Work out the finished part from the listing and answer in its coordinate system (mm). Face numbers are marked on the shaded views. A direction names the side the tool comes from. Coordinates: 2 decimals unless noted, no trailing zeros. Loops run counter-clockwise (first coordinate to the right, second up) from the corner with the lowest first, then second, coordinate; pieces in that order, holes last. Notation, with made-up numbers: (34, 20.25) - (91, 20.25) arc R26 ccw to (91, 57.25) - close; hole circle Ø11 at (4, 61). An arc over 180 degrees is marked (long way). Write each question's results on one line, items separated by ' | '. Start each with the question number.
Item 1: Consider probe 1 along Z at (x, y) = (11, -5); probe 2 along Z at (x, y) = (50.5, -19); probe 3 along Z at (x, y) = (7.5, -9.5). Determine where each line is inside the solid, lowest interval first. Write a range as [from, to].
Item 2: Each of these flat-tipped pins is pushed along its axis until it touches: pin 1 Ø5.5 at (x, y) = (8, -12) entering from -Z; pin 2 Ø6 at (x, y) = (28.5, 0.5) entering from +Z; pin 3 Ø4 at (y, z) = (-1, 0) entering from +X. Where does it stop, or does it pass through?
Item 3: A tool of negligible diameter and unlimited length cuts with its end or side. For the marked faces 4 and 5, from which of +Z, -Z, +X, -X, +Y, -Y can it reach the whole face along a straight path? Write none if from no direction.
Item 4: For a pull along X with two mould halves and no side action, classify the marked faces 1, 2 and 3 as +X half, -X half, draft (parallel to the pull), parting line (faces both ways), or undercut.
Item 5: Section A-A, the plane x = 18 is taken. Write down the section's boundary in (y, z).
from build123d import *

# Parameters (mm, degrees)
EXTRUDE_THIN1_DEPTH = 100
CUT_EXTRUDE2_DEPTH  = 33.5
FILLET1_R           = 3
SKETCH6_W           = 108.67085681690114
SKETCH6_H           = 17.87977423217149
CUT_EXTRUDE3_DEPTH  = 166
BOSS_EXTRUDE1_DEPTH = 10.5
CUT_EXTRUDE4_DEPTH  = 27.00000000000001
SKETCH11_R          = 1.749999999999997
CUT_EXTRUDE5_DEPTH  = 5
BOSS_EXTRUDE2_DEPTH = 7.500000000000001
CUT_EXTRUDE6_START  = -15.000000000000002
CUT_EXTRUDE6_DEPTH  = 15.000000000000002
FILLET3_R           = 2
CUT_EXTRUDE7_DEPTH  = 5.000000000000001
FILLET5_R           = 12


with BuildPart() as part:
    # Sketch1 → Extrude-Thin1 (new body)
    with BuildSketch(Plane(origin=(0, 0, 0), x_dir=(0, 0, -1), z_dir=(1, 0, 0))):
        with BuildLine():
            Line((44.99999999999999, -32), (45, -18.000000000000004))
            ThreePointArc((45, -18.000000000000004), (32.040658090715816, -6.957616725901104), (16.501342127994352, -3.94e-15))
            ThreePointArc((16.501342127994352, -3.94e-15), (-9.68e-15, 1.9727576042150758), (-16.501342127994352, 2.58e-15))
            ThreePointArc((-16.501342127994352, 2.58e-15), (-32.040658090715816, -6.957616725901083), (-45, -17.99999999999999))
            Line((-45, -17.99999999999999), (-45.00000000000001, -31.999999999999986))
            Line((-45.00000000000001, -31.999999999999986), (-48.00000000000001, -31.999999999999986))
            Line((-48.00000000000001, -31.999999999999986), (-48, -16.881858139762553))
            ThreePointArc((-48, -16.881858139762553), (-34.09998293164343, -4.712774745757805), (-17.2676846598946, 2.901081047578947))
            ThreePointArc((-17.2676846598946, 2.901081047578947), (-9.055e-14, 4.972757604215076), (17.26768465989443, 2.901081047578978))
            ThreePointArc((17.26768465989443, 2.901081047578978), (34.099982931643346, -4.71277474575777), (48, -16.881858139762553))
            Line((48, -16.881858139762553), (47.99999999999999, -32))
            Line((47.99999999999999, -32), (44.99999999999999, -32))
        make_face()
    extrude(amount=EXTRUDE_THIN1_DEPTH)

    # Sketch5 → Cut-Extrude2 (cut, symmetric)
    with BuildSketch(Plane(origin=(0, 0, 0), x_dir=(1, 0, 0), z_dir=(0, 1, 0))):
        with BuildLine():
            Line((74.78082212000585, 2.9999999999999996), (74.78082212000585, -3.0000000000000004))
            add(Edge.make_bspline(
                [(74.78082212000585, -3.0000000000000004), (97.6340902919286, -10.562952056895462), (100, -44)],
                knots=[0, 0, 0, 1, 1, 1], degree=2))
            Line((100, -44), (100, 44))
            add(Edge.make_bspline(
                [(74.78082212000585, 2.9999999999999996), (97.6340902919286, 10.562952056895462), (100, 44)],
                knots=[0, 0, 0, 1, 1, 1], degree=2))
        make_face()
    extrude(amount=CUT_EXTRUDE2_DEPTH, both=True, mode=Mode.SUBTRACT)

    # Fillet1
    fillet1_edges = [part.edges().sort_by_distance(p)[0] for p in [
        (50, -16.881858139762556, -48),
        (50, -16.88185813976255, 48),
        (74.78082212000585, 3.4097650316477264, 3.0000000000000004),
        (74.78082212000585, 3.4097650316477246, -2.9999999999999996),
        (46.32817175668929, 2.9010810475789732, -17.267684659894428),
        (46.328171756689336, 2.9010810475789484, 17.267684659894588),
    ]]
    fillet(fillet1_edges, radius=FILLET1_R)

    # Sketch6 → Cut-Extrude3 (cut)
    with BuildSketch(Plane(origin=(0, -2.379e-14, -48.00000000000001), x_dir=(-1, 0, 0), z_dir=(0, -5e-16, -1))):
        with Locations((-40.66457159154943, -32.93988711608573)):
            Rectangle(SKETCH6_W, SKETCH6_H)
    extrude(amount=-CUT_EXTRUDE3_DEPTH, mode=Mode.SUBTRACT)

    # Sketch8 → Boss-Extrude1 (add, symmetric)
    with BuildSketch(Plane.XY):
        Polygon((0, 1.9727576042150723), (-2.8489105039621805, -17.99999999999999), (7.1510894960378195, -17.99999999999999), (15, 1.972757604215074), align=None)
    extrude(amount=BOSS_EXTRUDE1_DEPTH, both=True)

    # Sketch10 → Cut-Extrude4 (cut)
    with BuildSketch(Plane.XY.offset(10.5)):
        with BuildLine():
            Line((-0.3489105039621806, -17.99999999999999), (3.9871579959635945, -17.99999999999999))
            ThreePointArc((3.9871579959635945, -17.99999999999999), (1.8191237460007066, -14.255159652410038), (-0.3489105039621806, -17.99999999999999))
        make_face()
    extrude(amount=-CUT_EXTRUDE4_DEPTH, mode=Mode.SUBTRACT)

    # Sketch11 → Cut-Extrude5 (cut)
    with BuildSketch(Plane(origin=(0, -2.379e-14, -48.00000000000001), x_dir=(-1, 0, 0), z_dir=(0, -5e-16, -1))):
        with Locations(Location((-95, -18.99999999999998, 0), (0, 0, 34.849904579))):
            Circle(SKETCH11_R)
    cut_extrude5 = extrude(amount=-CUT_EXTRUDE5_DEPTH, mode=Mode.SUBTRACT)

    # Mirror1: Cut-Extrude5 across plane
    add(cut_extrude5.mirror(Plane.XY), mode=Mode.SUBTRACT)

    # Sketch12 → Boss-Extrude2 (add, symmetric)
    with BuildSketch(Plane.XY):
        Polygon((74.78082212000585, 1.9727576042150723), (74.78082212000585, -15.901753636370586), (83.21987044067507, -15.901753636370586), (83.21987044067507, -19.589110757152636), (67.6773818593807, -19.589110757152636), (67.6773818593807, 1.9727576042150723), align=None)
    extrude(amount=BOSS_EXTRUDE2_DEPTH, both=True)

    # Sketch13 → Cut-Extrude6 (cut)
    with BuildSketch(Plane(origin=(74.78082212000585, 0, 0), x_dir=(0, 0, -1), z_dir=(1, 0, 0)).offset(CUT_EXTRUDE6_START)):
        with BuildLine():
            Line((-7.500000000000001, 1.569812139590343), (-7.499999999999999, -15.901753636370586))
            Line((-7.499999999999999, -15.901753636370586), (-3.7049771024193907, -15.901753636370586))
            Line((-3.7049771024193907, -15.901753636370586), (-3.7049771024193907, 1.8746398726529334))
            ThreePointArc((-3.7049771024193907, 1.8746398726529334), (-5.604561352429517, 1.748031821138369), (-7.500000000000001, 1.569812139590343))
        make_face()
        with BuildLine():
            Line((7.499999999999999, -15.901753636370586), (3.7049771024193907, -15.901753636370586))
            Line((3.7049771024193907, -15.901753636370586), (3.7049771024193907, 1.8746398726529334))
            ThreePointArc((3.7049771024193907, 1.8746398726529334), (5.6045613524295295, 1.7480318211384258), (7.500000000000001, 1.569812139590343))
            Line((7.500000000000001, 1.569812139590343), (7.499999999999999, -15.901753636370586))
        make_face()
    extrude(amount=CUT_EXTRUDE6_DEPTH, mode=Mode.SUBTRACT)

    # Fillet3
    fillet3_edges = [part.edges().sort_by_distance(p)[0] for p in [
        (75.44862615002788, -15.901753636370586, -7.5),
        (83.21987044067507, -15.901753636370586, 0),
        (75.44862615002788, -15.901753636370586, 7.5),
        (67.6773818593807, -7.013556881858825, -3.7049771024193907),
        (67.6773818593807, -7.013556881858825, 3.7049771024193907),
        (74.78082212000585, -7.013556881858825, 3.7049771024193907),
        (74.78082212000585, -7.013556881858825, -3.7049771024193907),
    ]]
    fillet(fillet3_edges, radius=FILLET3_R)

    # Sketch15 → Cut-Extrude7 (cut)
    with BuildSketch(Plane(origin=(0, -2.379e-14, -48.00000000000001), x_dir=(-1, 0, 0), z_dir=(0, -5e-16, -1))):
        Polygon((-95, -23.99999999999998), (0, -18.860125054588586), (0, -26.572046869734645), align=None)
    cut_extrude7 = extrude(amount=-CUT_EXTRUDE7_DEPTH, mode=Mode.SUBTRACT)

    # Mirror2: Cut-Extrude7 across plane
    add(cut_extrude7.mirror(Plane.XY), mode=Mode.SUBTRACT)

    # Fillet5
    # the kernel refuses this fillet: 12 mm, written as the material it takes off along each edge
    with BuildSketch(Plane(origin=(0, -18.860125054588625, 76.42075806632201), x_dir=(0, 1, 5e-16), z_dir=(0, 5e-16, -1))) as fillet5_piece_1:
        with BuildLine():
            CenterArc((FILLET5_R * 0.947358602211, FILLET5_R), FILLET5_R, 183.09690836649892, 86.90309163350105)
            Line((-FILLET5_R * 0.0511809847104, FILLET5_R * 0.945975067318), (0, 0))
            Line((0, 0), (FILLET5_R * 0.947358602211, 0))
        make_face()
    extrude(amount=59.841516132644024, mode=Mode.SUBTRACT)
    with BuildSketch(Plane(origin=(0, -18.860125054588625, -76.42075806632201), x_dir=(0, 1, -5e-16), z_dir=(0, 5e-16, 1))) as fillet5_piece_2:
        with BuildLine():
            CenterArc((FILLET5_R * 0.947358602211, -FILLET5_R), FILLET5_R, 90, 86.90309163350108)
            Line((-FILLET5_R * 0.0511809847104, -FILLET5_R * 0.945975067318), (0, 0))
            Line((0, 0), (FILLET5_R * 0.947358602211, 0))
        make_face()
    extrude(amount=59.841516132644024, mode=Mode.SUBTRACT)


solid = part.part
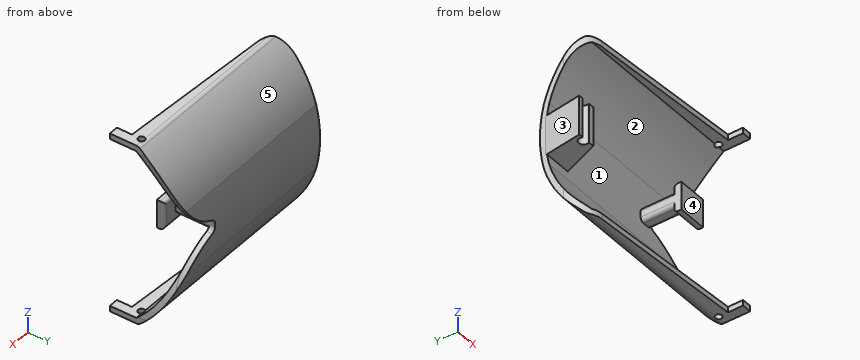
Answer key:
1) probe 1: z = [-34.54, -28.71], [-10.5, 10.5], [28.71, 34.54] | probe 2: z = [-48, -45], [45, 48] | probe 3: z = [-40.58, -35.75], [-10.5, 10.5], [35.75, 40.58]
2) pin 1: stops at z = -46.1 | pin 2: stops at z = 30.39 | pin 3: stops at x = 74.78
3) face 4: +X, -X, -Y | face 5: +Z, +X, -X, +Y
4) face 1: undercut | face 2: draft | face 3: -X half
5) outline: (-19.83, -48) - (-18, -48) arc R3 ccw to (-16.02, -47.25) arc R63 ccw to (2.9, -17.27) arc R73 ccw to (2.9, 17.27) arc R63 ccw to (-16.02, 47.25) arc R3 ccw to (-18, 48) - (-19.83, 48) - (-19.83, 45) - (-18, 45) arc R60 cw to (0, 16.5) arc R70 cw to (0, -16.5) arc R60 cw to (-18, -45) - (-19.83, -45) - close
